The model under review builds one solid part; all positions refer to its coordinate system, in mm. Face numbers are marked on the shaded views. A direction names the side the tool comes from. Coordinates: 2 decimals unless noted, no trailing zeros. Order: outer loops, then holes, each group sorted by start corner. A loop starts at its lowest first (then second) coordinate and runs counter-clockwise, first axis right, second up. Notation, with made-up numbers: (6, 70.25) -> (65, 70.25) arc R16 cw to (65, 75.25) -> close; hole circle Ø3 at (0, 44.25). An arc over 180 degrees is marked (long way). Use one line per item in the form item = value.
Autodesk Inventor part; units mm, degrees
ref_plane "YZ Plane" through (0, 0, 0) normal (1, 0, 0) x (0, 1, 0)
ref_plane "XZ Plane" through (0, 0, 0) normal (0, 1, 0) x (-1, 0, 0)
ref_plane "XY Plane" through (0, 0, 0) normal (0, 0, 1) x (1, 0, 0)
sketch "Эскиз1" plane through (0, 0, 0) normal (1, 0, 0) x (0, 1, 0)
  line L0 (0, 0) -> (15, 0)
  line L1 (15, 0) -> (15, -20)
  line L2 (15, -20) -> (0, -20)
  line L3 (0, -20) -> (0, 0)
  dimension "d0" = 15
  dimension "d1" = 20
extrude "Выдавливание1" add sketch "Эскиз1" along normal blind 1
sketch "Эскиз2" plane through (1, 0, 0) normal (1, 0, 0) x (0, 0, -1)
  line L0 (0, 0) -> (20, 0)
  line L1 (20, 15) -> (0, 15)
  line L2 (0, 0) -> (18.5, 0)
  line L3 (18.5, 0) -> (18.5, 15)
  line L4 (18.5, 15) -> (0, 15)
  line L5 (0, 15) -> (0, 0)
  point P0 (0, 15)
  dimension "d4" = 18.5
extrude "Выдавливание2" add sketch "Эскиз2" along normal blind 5
sketch "Эскиз3" plane through (0, 0, 0) normal (-1, 0, 0) x (0, 0, 1)
  circle A0 centre (-10, 7.5) radius 3
  line L0 (-20, 0) -> (-20, 15)
  line L1 (-20, 15) -> (0, 15)
  point P0 (0, 0)
  dimension "d7" = 6
  dimension "d8" = 10
  dimension "d9" = 7.5
extrude "Выдавливание3" cut sketch "Эскиз3" against normal blind 10
fillet "Сопряжение1" radius 1 1 edges at (1, 7.5, -18.5)
fillet "Сопряжение2" radius 2 2 edges at (3, 0, 0) (3, 15, 0)
properties part number "CableHolder"
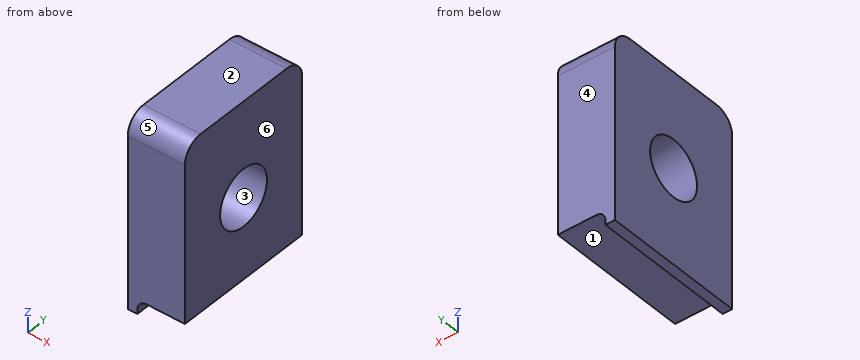
Item 1: Clearance check with flat-ended pins moving along their axes: pin 1 (0.6 mm diameter, centred on y = 8.5, z = -20, fed in from +X); pin 2 (1.2 mm diameter, centred on x = 4, y = 9.5, fed in from -Z). State where each tip first meets the part, or that it passes through.
Results found:
pin_1 = 1
pin_2 = -18.5
Item 2: To check wall thickness, follow L1, parallel to Y at x = 4.3, z = -10; L2, parallel to Z at x = 1.2, y = 6.75; L3, parallel to Z at x = 5.2, y = 10.25. State the ranges of each line that lie inside material, in increasing order. Write a range as from..to.
Results found:
L1 = 0..4.5, 10.5..15
L2 = -18.9..-12.9, -7.1..0
L3 = -18.5..-11.2, -8.8..0
Item 3: We need section A-A (z = -10). Write out the cut boundary in (x, y), plus the area to 3 significant figures.
Results found:
outline = (0, 0) -> (6, 0) -> (6, 4.5) -> (0, 4.5) -> close; (0, 10.5) -> (6, 10.5) -> (6, 15) -> (0, 15) -> close
area = 54.0 mm²
Item 4: We need section B-B (y = 7.5). Write out the cut boundary in (x, z), plus the area to 3 significant figures.
Results found:
outline = (0, -20) -> (1, -20) -> (1, -19.5) arc R1 cw to (2, -18.5) -> (6, -18.5) -> (6, -13) -> (0, -13) -> close; (0, -7) -> (6, -7) -> (6, 0) -> (0, 0) -> close
area = 76.7 mm²
Item 5: We need section D-D (y = 14). Write out the cut boundary in (x, z).
Results found:
outline = (0, -20) -> (1, -20) -> (1, -19.5) arc R1 cw to (2, -18.5) -> (6, -18.5) -> (6, -0.27) -> (0, -0.27) -> close
Item 6: Tool access review of the marked faces 1 and 2: name each direction out of +Z, -Z, +X, -X, +Y, -Y from which nothing blocks a thin tool from reaching the whole face with its end or side.
Results found:
face_1 = -Z, +X, +Y, -Y
face_2 = +Z, +X, -X, +Y, -Y
Item 7: We need section C-C (x = 5.5). Write out the cut boundary in (y, z).
Results found:
outline = (0, -18.5) -> (15, -18.5) -> (15, -2) arc R2 ccw to (13, 0) -> (2, 0) arc R2 ccw to (0, -2) -> close; hole circle Ø6 at (7.5, -10)
Item 8: Draft analysis for pull direction Y (two halves, no side actions). For the marked faces 3, 4, 5 and 6, state which applies: released by +Y, released by -Y, zero draft, split by the parting line, or undercut.
Results found:
face_3 = undercut
face_4 = released by +Y
face_5 = released by -Y
face_6 = zero draft
